```python
from build123d import *

# Parameters (mm, degrees)
SKETCH1_W                  = 180
SKETCH1_H                  = 140
BOSS_EXTRUDE1_DEPTH        = 22
CUT_EXTRUDE1_DEPTH         = 17
FILLET1_R                  = 2
FILLET2_R                  = 13
CUT_EXTRUDE2_DEPTH         = 4.2
FILLET3_R                  = 10
F_11_0_11_DIAMETER_HOLE1_D = 11
M6_CLEARANCE_HOLE1_D       = 6.4
SKETCH11_R                 = 5.5
CUT_EXTRUDE6_DEPTH         = 7


with BuildPart() as part:
    # Sketch1 → Boss-Extrude1 (new body)
    with BuildSketch(Plane.XY):
        Rectangle(SKETCH1_W, SKETCH1_H)
    extrude(amount=BOSS_EXTRUDE1_DEPTH)

    # Sketch2 → Cut-Extrude1 (cut)
    with BuildSketch(Plane.XY.offset(22)):
        Polygon((-66.5, 61.5), (66.5, 61.5), (66.5, 31.5), (82.5, 31.5), (82.5, -31.5), (66.5, -31.5), (66.5, -61.5), (-66.5, -61.5), (-66.5, -31.5), (-82.5, -31.5), (-82.5, 31.5), (-66.5, 31.5), align=None)
    extrude(amount=-CUT_EXTRUDE1_DEPTH, mode=Mode.SUBTRACT)

    # Fillet1
    fillet1_edges = [part.edges().sort_by_distance(p)[0] for p in [
        (-66.5, 61.5, 13.5),
        (66.5, 61.5, 13.5),
        (82.5, 31.5, 13.5),
        (82.5, -31.5, 13.5),
        (66.5, -61.5, 13.5),
        (-66.5, -61.5, 13.5),
        (-82.5, -31.5, 13.5),
        (-82.5, 31.5, 13.5),
    ]]
    fillet(fillet1_edges, radius=FILLET1_R)

    # Fillet2
    fillet2_edges = [part.edges().sort_by_distance(p)[0] for p in [
        (-66.5, 31.5, 13.5),
        (66.5, 31.5, 13.5),
        (66.5, -31.5, 13.5),
        (-66.5, -31.5, 13.5),
    ]]
    fillet(fillet2_edges, radius=FILLET2_R)

    # Sketch3 → Cut-Extrude2 (cut)
    with BuildSketch(Plane.XY.offset(22)):
        with BuildLine():
            Line((-72, 59.5), (-72, 44.5))
            ThreePointArc((-72, 44.5), (-74.196699141, 39.196699141), (-79.5, 37))
            Line((-79.5, 37), (-80.5, 37))
            ThreePointArc((-80.5, 37), (-85.803300859, 34.803300859), (-88, 29.5))
            Line((-88, 29.5), (-88, -29.5))
            ThreePointArc((-88, -29.5), (-85.803300859, -34.803300859), (-80.5, -37))
            Line((-80.5, -37), (-79.5, -37))
            ThreePointArc((-79.5, -37), (-74.196699141, -39.196699141), (-72, -44.5))
            Line((-72, -44.5), (-72, -59.5))
            ThreePointArc((-72, -59.5), (-69.803300859, -64.803300859), (-64.5, -67))
            Line((-64.5, -67), (64.5, -67))
            ThreePointArc((64.5, -67), (69.803300859, -64.803300859), (72, -59.5))
            Line((72, -59.5), (72, -44.5))
            ThreePointArc((72, -44.5), (74.196699141, -39.196699141), (79.5, -37))
            Line((79.5, -37), (80.5, -37))
            ThreePointArc((80.5, -37), (85.803300859, -34.803300859), (88, -29.5))
            Line((88, -29.5), (88, 29.5))
            ThreePointArc((88, 29.5), (85.803300859, 34.803300859), (80.5, 37))
            Line((80.5, 37), (79.5, 37))
            ThreePointArc((79.5, 37), (74.196699141, 39.196699141), (72, 44.5))
            Line((72, 44.5), (72, 59.5))
            ThreePointArc((72, 59.5), (69.803300859, 64.803300859), (64.5, 67))
            Line((64.5, 67), (-64.5, 67))
            ThreePointArc((-64.5, 67), (-69.803300859, 64.803300859), (-72, 59.5))
        make_face()
        with BuildLine():
            Line((-80.5, -33.5), (-79.5, -33.5))
            ThreePointArc((-79.5, -33.5), (-71.721825407, -36.721825407), (-68.5, -44.5))
            Line((-68.5, -44.5), (-68.5, -59.5))
            ThreePointArc((-68.5, -59.5), (-67.328427125, -62.328427125), (-64.5, -63.5))
            Line((-64.5, -63.5), (64.5, -63.5))
            ThreePointArc((64.5, -63.5), (67.328427125, -62.328427125), (68.5, -59.5))
            Line((68.5, -59.5), (68.5, -44.5))
            ThreePointArc((68.5, -44.5), (71.721825407, -36.721825407), (79.5, -33.5))
            Line((79.5, -33.5), (80.5, -33.5))
            ThreePointArc((80.5, -33.5), (83.328427125, -32.328427125), (84.5, -29.5))
            Line((84.5, -29.5), (84.5, 29.5))
            ThreePointArc((84.5, 29.5), (83.328427125, 32.328427125), (80.5, 33.5))
            Line((80.5, 33.5), (79.5, 33.5))
            ThreePointArc((79.5, 33.5), (71.721825407, 36.721825407), (68.5, 44.5))
            Line((68.5, 44.5), (68.5, 59.5))
            ThreePointArc((68.5, 59.5), (67.328427125, 62.328427125), (64.5, 63.5))
            Line((64.5, 63.5), (-64.5, 63.5))
            ThreePointArc((-64.5, 63.5), (-67.328427125, 62.328427125), (-68.5, 59.5))
            Line((-68.5, 59.5), (-68.5, 44.5))
            ThreePointArc((-68.5, 44.5), (-71.721825407, 36.721825407), (-79.5, 33.5))
            Line((-79.5, 33.5), (-80.5, 33.5))
            ThreePointArc((-80.5, 33.5), (-83.328427125, 32.328427125), (-84.5, 29.5))
            Line((-84.5, 29.5), (-84.5, -29.5))
            ThreePointArc((-84.5, -29.5), (-83.328427125, -32.328427125), (-80.5, -33.5))
        make_face(mode=Mode.SUBTRACT)
    extrude(amount=-CUT_EXTRUDE2_DEPTH, mode=Mode.SUBTRACT)

    # Fillet3
    fillet3_edges = [part.edges().sort_by_distance(p)[0] for p in [
        (-90, 70, 11),
        (90, 70, 11),
        (90, -70, 11),
        (-90, -70, 11),
    ]]
    fillet(fillet3_edges, radius=FILLET3_R)

    # Ø11.0 (11) Diameter Hole1 (through all)
    with Locations(Plane.XY.offset(22)):
        with Locations((-80, 45), (-80, -45), (80, -45), (80, 45)):
            Hole(F_11_0_11_DIAMETER_HOLE1_D / 2)

    # M6 Clearance Hole1 (through all)
    with Locations(Plane.XY.offset(22)):
        with Locations((-80, 60), (-80, -60), (80, -60), (80, 60)):
            Hole(M6_CLEARANCE_HOLE1_D / 2)

    # Sketch11 → Cut-Extrude6 (cut)
    with BuildSketch(Plane(origin=(0, 0, 0), x_dir=(-1, 0, 0), z_dir=(0, 0, -1))):
        with Locations((-80, 60)):
            Circle(SKETCH11_R)
        with Locations((-80, -60)):
            Circle(SKETCH11_R)
        with Locations((80, -60)):
            Circle(SKETCH11_R)
        with Locations((80, 60)):
            Circle(SKETCH11_R)
    extrude(amount=-CUT_EXTRUDE6_DEPTH, mode=Mode.SUBTRACT)


solid = part.part
```
The listing builds one solid part. Answer for the finished solid, in the listing's coordinates (mm). A direction names the side the tool comes from. Coordinates: 2 decimals unless noted, no trailing zeros. Write each loop counter-clockwise with the first axis right and the second up, starting at its lowest first coordinate (ties: lowest second). Pieces come first, ordered by that corner, then holes. Notation, with made-up numbers: (50.25, -31) - (59.25, -31) arc R10 ccw to (59.25, -19) - close; hole circle Ø5 at (45, -20.5). An arc over 180 degrees is marked (long way). Return JSON: item names as keys, results as strings. Group by question number.
1. Determine the mould class of faces 4 (the cylindrical face through (85.495, -44.758, 10.846)), 5 (the cylindrical face through (-87.15, -66.99, 11.15)) for opening direction X: released by +X, released by -X, zero draft, split by the parting line, or undercut.
2. A cutting plane is placed at B-B, the plane x = -33.5. Determine the outline of the cut face in (y, z).
3. A cutting plane is placed at D-D, the plane z = 20. Give the number of separate pieces and of enclosed holes in the cut face, plus the area to 3 significant figures.
4. Straight lines are drawn through the part: L1, parallel to X at y = -56, z = 20.25; L2, parallel to Y at x = 80, z = 11; L3, parallel to Y at x = -23.5, z = 14.25. For each, find the intervals that lie inside material, in ascending order.
5. Which of the six approach directions +Z, -Z, +X, -X, +Y, -Y give full straight-line access (tool end or side, diameter ignored) to faces 1 (the cylindrical face through (85.495, -59.758, 3.451)), 2 (the flat face through (-68.5, -52, 20)), 3 (the cylindrical face through (85.495, 45.242, 10.846))?
6. A cutting plane is placed at C-C, the plane y = -42.5. Determine the outline of the cut face in (x, z), plus the area to 3 significant figures.
7. Given pin 1 (10 mm diameter, centred on x = -80, y = 45, fed in from +Z); pin 2 (5.5 mm diameter, centred on x = -80, y = 62, fed in from -Z), each flat-ended and moving along its own axis, determine where each tip first touches the part or whether it passes through.
8. A cutting plane is placed at A-A, the plane y = 2. Determine the outline of the cut face in (x, z).
Ans:
{
 "1": {"face 4": "undercut", "face 5": "released by -X"},
 "2": {"outline": "(-70, 0) - (70, 0) - (70, 22) - (67, 22) - (67, 17.8) - (63.5, 17.8) - (63.5, 22) - (61.5, 22) - (61.5, 5) - (-61.5, 5) - (-61.5, 22) - (-63.5, 22) - (-63.5, 17.8) - (-67, 17.8) - (-67, 22) - (-70, 22) - close"},
 "3": {"separate pieces": "2", "enclosed holes": "10", "area": "4,100 mm²"},
 "4": {"L1": "-90 to -72, -68.5 to -66.5, 66.5 to 68.5, 72 to 90", "L2": "-70 to -63.2, -56.8 to -50.5, -39.5 to -31.5, 31.5 to 39.5, 50.5 to 56.8, 63.2 to 70", "L3": "-70 to -61.5, 61.5 to 70"},
 "5": {"face 1": "-Z", "face 2": "+Z", "face 3": "+Z, -Z"},
 "6": {"outline": "(-90, 0) - (-84.9, 0) - (-84.9, 22) - (-90, 22) - close; (-75.1, 0) - (75.1, 0) - (75.1, 22) - (72.27, 22) - (72.27, 17.8) - (68.68, 17.8) - (68.68, 22) - (66.65, 22) - (66.65, 5) - (-66.65, 5) - (-66.65, 22) - (-68.68, 22) - (-68.68, 17.8) - (-72.27, 17.8) - (-72.27, 22) - (-75.1, 22) - close; (84.9, 0) - (90, 0) - (90, 22) - (84.9, 22) - close", "area": "1,230 mm²"},
 "7": {"pin 1": "through", "pin 2": "z = 7"},
 "8": {"outline": "(-90, 0) - (90, 0) - (90, 22) - (88, 22) - (88, 17.8) - (84.5, 17.8) - (84.5, 22) - (82.5, 22) - (82.5, 5) - (-82.5, 5) - (-82.5, 22) - (-84.5, 22) - (-84.5, 17.8) - (-88, 17.8) - (-88, 22) - (-90, 22) - close"}
}
